Job drawing, mm, ordinate dimensions from the low corner. One solid piece. A direction names the side the tool comes from. Round coordinates to 2 decimals unless told otherwise and drop trailing zeros. Order: outer loops, then holes, each group sorted by start corner. A loop starts at its lowest first (then second) coordinate and runs counter-clockwise, first axis right, second up. Notation, with made-up numbers: (37.5, 58) -> (57.5, 58) arc R12 ccw to (57.5, 71) -> close; hole circle Ø10 at (-40, 46.25). An arc over 180 degrees is marked (long way). Return JSON: item names as keys, results as strings. Group by question number.
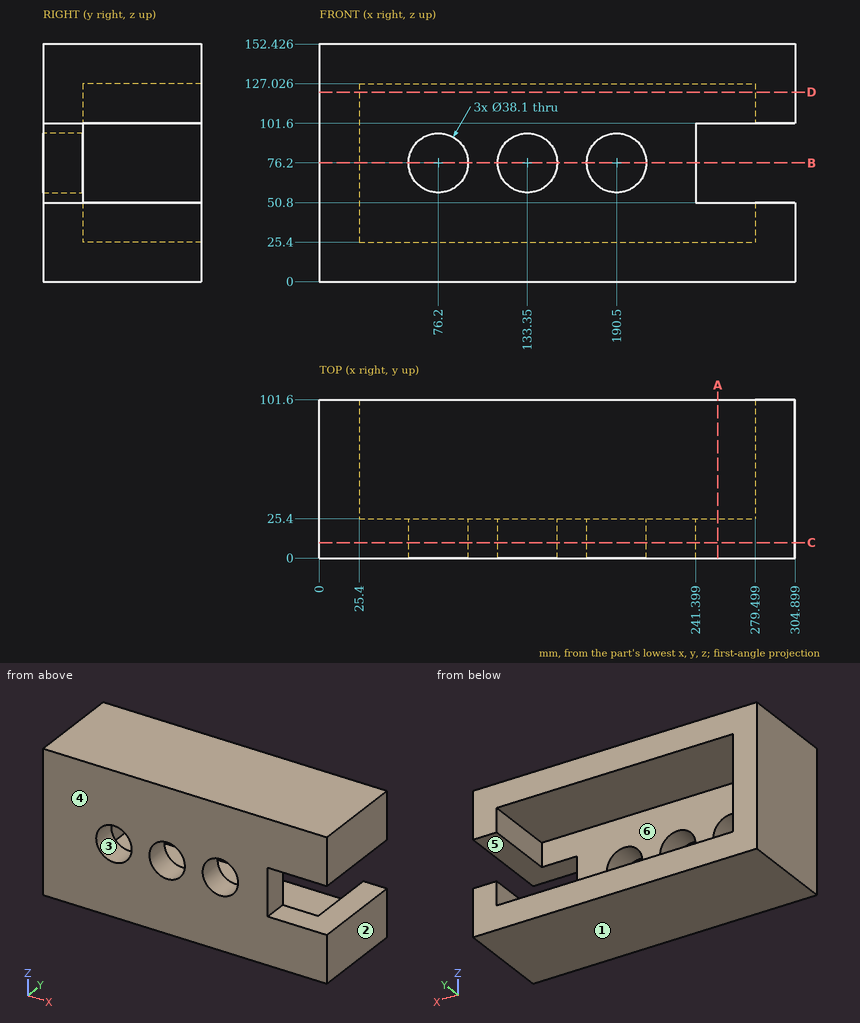
(1) Pin check, flat tips, straight feed: P1, Ø12.5, axis at y = 10, z = 71.5, coming from the +X side; P2, Ø23, axis at y = 70, z = 66, coming from the +X side. Stop position of each tip, or through.
(2) Saw through at C-C, the plane y = 10. List the corners of the cut face in (x, z).
(3) Saw through at B-B, the plane z = 76.2. List the corners of the cut face in (x, y).
(4) Saw through at A-A, the plane x = 255.5. List the corners of the cut face in (y, z).
(5) Mould opens along Z. For the marked faces 1, 2 and 3 say: pulls with the +Z half, pulls with the -Z half, needs draft (parallel to the pull), parting line crosses it, or undercut.
(6) Saw through at D-D, the plane z = 121.5. List the corners of the cut face in (x, y).
(7) Probe L1, parallel to X at y = 11, z = 76.2; L2, parallel to Z at x = 292, y = 57; L3, parallel to Z at x = 165, y = 44.5. List the from-to ranges inside material, lowest first. Write a range as [from, to].
(8) Tool access for the marked faces 4, 5 and 6: list every direction of +Z, -Z, +X, -X, +Y, -Y with a clear straight run to the whole face (end or side of a thin tool).
Results are:
{
 "1": {"P1": "stops at x = 241.4", "P2": "stops at x = 25.4"},
 "2": {"outline": "(0, 0) -> (304.9, 0) -> (304.9, 50.8) -> (241.4, 50.8) -> (241.4, 101.6) -> (304.9, 101.6) -> (304.9, 152.43) -> (0, 152.43) -> close; hole circle Ø38.1 at (76.2, 76.2); hole circle Ø38.1 at (133.35, 76.2); hole circle Ø38.1 at (190.5, 76.2)"},
 "3": {"outline": "(0, 0) -> (57.15, 0) -> (57.15, 25.4) -> (25.4, 25.4) -> (25.4, 101.6) -> (0, 101.6) -> close; (95.25, 0) -> (114.3, 0) -> (114.3, 25.4) -> (95.25, 25.4) -> close; (152.4, 0) -> (171.45, 0) -> (171.45, 25.4) -> (152.4, 25.4) -> close; (209.55, 0) -> (241.4, 0) -> (241.4, 25.4) -> (209.55, 25.4) -> close"},
 "4": {"outline": "(0, 0) -> (101.6, 0) -> (101.6, 25.4) -> (25.4, 25.4) -> (25.4, 50.8) -> (0, 50.8) -> close; (0, 101.6) -> (25.4, 101.6) -> (25.4, 127.03) -> (101.6, 127.03) -> (101.6, 152.43) -> (0, 152.43) -> close"},
 "5": {"face 1": "pulls with the -Z half", "face 2": "needs draft", "face 3": "undercut"},
 "6": {"outline": "(0, 0) -> (304.9, 0) -> (304.9, 101.6) -> (279.5, 101.6) -> (279.5, 25.4) -> (25.4, 25.4) -> (25.4, 101.6) -> (0, 101.6) -> close"},
 "7": {"L1": "x = [0, 57.15], [95.25, 114.3], [152.4, 171.45], [209.55, 241.4]", "L2": "z = [0, 50.8], [101.6, 152.43]", "L3": "z = [0, 25.4], [127.03, 152.43]"},
 "8": {"face 4": "+Z, -Z, +X, -X, -Y", "face 5": "+X, +Y, -Y", "face 6": "+Y"}
}
